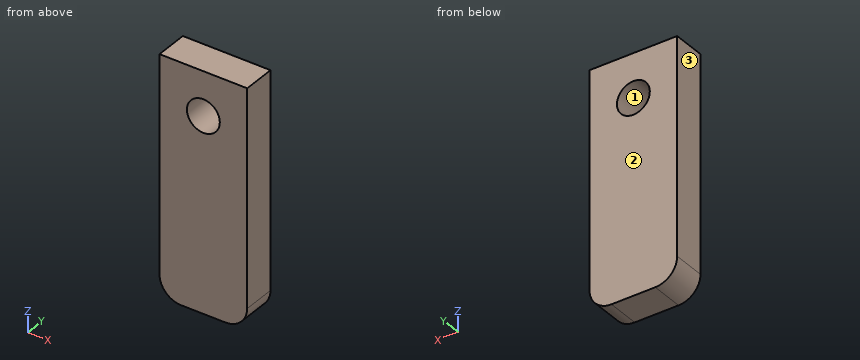
```python
from build123d import *

# Parameters (mm, degrees)
SKETCH1_R           = 1.5
BOSS_EXTRUDE1_DEPTH = 3


with BuildPart() as part:
    # Sketch1 → Boss-Extrude1 (new body)
    with BuildSketch(Plane(origin=(0, 0, 0), x_dir=(1, 0, 0), z_dir=(0, 1, 0))):
        with BuildLine():
            Line((4, -10.823913854), (-4, -10.823913854))
            Line((-4, -10.823913854), (-4, 8.823913854))
            ThreePointArc((-4, 8.823913854), (-3.414213562, 10.238127416), (-2, 10.823913854))
            Line((-2, 10.823913854), (2, 10.823913854))
            ThreePointArc((2, 10.823913854), (3.414213562, 10.238127416), (4, 8.823913854))
            Line((4, 8.823913854), (4, -10.823913854))
        make_face()
        with Locations(Location((0, -6.823913854, 0), (0, 0, 270))):
            Circle(SKETCH1_R, mode=Mode.SUBTRACT)
    extrude(amount=BOSS_EXTRUDE1_DEPTH)


solid = part.part
```
Geometry: final body of the model. Coordinates: model frame, mm. Face numbers are marked on the shaded views. Coordinates: 2 decimals unless noted, no trailing zeros. Write each loop counter-clockwise with the first axis right and the second up, starting at its lowest first coordinate (ties: lowest second). Pieces come first, ordered by that corner, then holes. Notation, with made-up numbers: M 48.25,0 L 66.25,0 A12 ccw 66.25,6 Z; hole C 43,-14.75 d10. An arc over 180 degrees is marked long. Answer as CSV lines item,"result". Start each with the question number.
Q1. Cut plane B-B on x = 0. Return the cut outline in (y, z), then the cut area to 3 significant figures.
Q2. Cut plane A-A on y = 1. Return the cut outline in (x, z).
Q3. Pin query (flat end, axial travel): P1, Ø3.5, axis at x = 0, z = 6.82, coming from the -Y side. Return the tip coordinate at first contact, or that it passes through.
Q4. Mould query, pull axis X, two halves, no side actions, for the marked faces 1, 2 and 3. Classes: released by +X, released by -X, zero draft, split by the parting line, or undercut.
Q5. Cut plane D-D on x = -3.5. Return the cut outline in (y, z), then the cut area to 3 significant figures.
Q6. Line query: line 1 (Z direction, x = -0.5, y = 1.55); line 2 (X direction, y = 1.45, z = 6.5); line 3 (Z direction, x = 1.25, y = 0.1). Output: solid intervals per line, ascending. Write a range as from..to.
Q7. Cut plane C-C on x = 1. Return the cut outline in (y, z).
Findings below:
1,outline,"M 0,-10.82 L 3,-10.82 L 3,5.32 L 0,5.32 Z; M 0,8.32 L 3,8.32 L 3,10.82 L 0,10.82 Z"
1,area,"55.9 mm2"
2,outline,"M -4,-8.82 A2 ccw -2,-10.82 L 2,-10.82 A2 ccw 4,-8.82 L 4,10.82 L -4,10.82 Z; hole C 0,6.82 d3"
3,P1,"stops at y = 0"
4,face 1,"undercut"
4,face 2,"zero draft"
4,face 3,"released by -X"
5,outline,"M 0,-10.15 L 3,-10.15 L 3,10.82 L 0,10.82 Z"
5,area,"62.9 mm2"
6,line 1,"z = -10.82..5.41, 8.24..10.82"
6,line 2,"x = -4..-1.46, 1.46..4"
6,line 3,"z = -10.82..5.99, 7.65..10.82"
7,outline,"M 0,-10.82 L 3,-10.82 L 3,5.71 L 0,5.71 Z; M 0,7.94 L 3,7.94 L 3,10.82 L 0,10.82 Z"
